```python
from build123d import *

# Parameters (mm, degrees)
F0_R     = 9.525
F1_DEPTH = 3.175


with BuildPart() as f1:
    # F0 (on Top) → F1 (new body)
    with BuildSketch(Plane.XY):
        Polygon((-2.000947, 38.180346), (-7.849032, 24.156836), (-20.823044, 32.064676), (-18.875879, 16.995917), (-34.065623, 17.357302), (-24.844949, 5.280957), (-38.180346, -2.000947), (-24.156836, -7.849032), (-32.064676, -20.823044), (-16.995917, -18.875879), (-17.357302, -34.065623), (-5.280957, -24.844949), (2.000947, -38.180346), (7.849032, -24.156836), (20.823044, -32.064676), (18.875879, -16.995917), (34.065623, -17.357302), (24.844949, -5.280957), (38.180346, 2.000947), (24.156836, 7.849032), (32.064676, 20.823044), (16.995917, 18.875879), (17.357302, 34.065623), (5.280957, 24.844949), align=None)
        Circle(F0_R, mode=Mode.SUBTRACT)
    extrude(amount=F1_DEPTH)


solid = f1.part
```
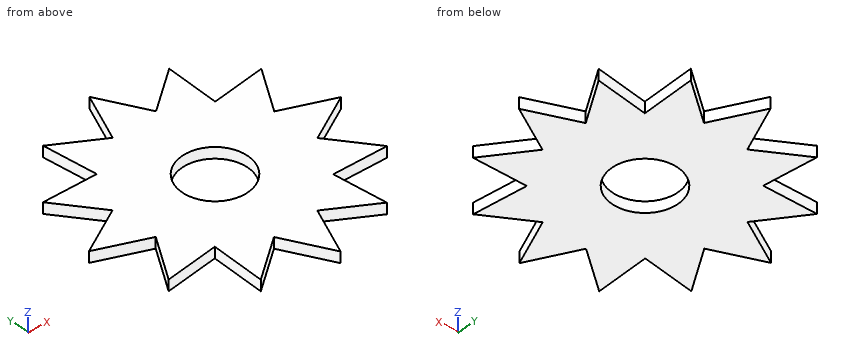
Input: part model. Units: mm. Frame: model coordinates. Coordinates: 2 decimals unless noted, no trailing zeros. Loops run counter-clockwise (first coordinate to the right, second up) from the corner with the lowest first, then second, coordinate; pieces in that order, holes last.
Q1. Section A-A, the plane z = 1.55. Return the cut outline in (x, y) (3 decimals), and give its area (3 significant figures).
Results are:
outline: (-38.18, -2.001) - (-24.157, -7.849) - (-32.065, -20.823) - (-16.996, -18.876) - (-17.357, -34.066) - (-5.281, -24.845) - (2.001, -38.18) - (7.849, -24.157) - (20.823, -32.065) - (18.876, -16.996) - (34.066, -17.357) - (24.845, -5.281) - (38.18, 2.001) - (24.157, 7.849) - (32.065, 20.823) - (16.996, 18.876) - (17.357, 34.066) - (5.281, 24.845) - (-2.001, 38.18) - (-7.849, 24.157) - (-20.823, 32.065) - (-18.876, 16.996) - (-34.066, 17.357) - (-24.845, 5.281) - close; hole circle Ø19.05 at (0, 0)
area: 2,730 mm2
Q2. Section D-D, the plane y = 26. Return the cut outline in (x, z) (3 decimals).
Results are:
outline: (-20.039, 0) - (-10.873, 0) - (-10.873, 3.175) - (-20.039, 3.175) - close; (-7.08, 0) - (4.65, 0) - (4.65, 3.175) - (-7.08, 3.175) - close; (6.794, 0) - (17.165, 0) - (17.165, 3.175) - (6.794, 3.175) - close
Q3. Contact query for flat-ended pins moving along their axis: pin 1 (1.5 mm diameter, centred on y = -11.5, z = 1.5, fed in from -X); pin 2 (1.5 mm diameter, centred on y = -21.5, z = 2, fed in from +X); pin 3 (1 mm diameter, centred on x = -0.5, z = 1, fed in from +Y). Output: stop coordinate, or through.
Results are:
pin 1: stops at x = -26.84
pin 2: stops at x = 19.55
pin 3: stops at y = 36.35
Q4. Section B-B, the plane x = 0. Return the cut outline in (y, z) (3 decimals).
Results are:
outline: (-34.516, 0) - (-9.525, 0) - (-9.525, 3.175) - (-34.516, 3.175) - close; (9.525, 0) - (34.516, 0) - (34.516, 3.175) - (9.525, 3.175) - close
Q5. Line query: line 1 along Y through (x, z) = (-25, 0.35); line 2 along X through (y, z) = (31.5, 0.8); line 3 along Y through (x, z) = (8.5, 2.8). Output: solid intervals per line, ascending.
Results are:
line 1: y = -19.91 to -9.23, -7.5 to 5.2, 5.48 to 17.14
line 2: x = -20.75 to -19.9, -4.79 to 1.65, 14 to 17.3
line 3: y = -24.55 to -4.3, 4.3 to 27.3
